Geometry check sheet. Reference: the model listing, model coordinates, mm. A direction names the side the tool comes from. Give positions to 0.01 mm unless a question says otherwise; leave off trailing zeros. Order: outer loops, then holes, each group sorted by start corner. A loop starts at its lowest first (then second) coordinate and runs counter-clockwise, first axis right, second up.
Autodesk Inventor part; units mm, degrees
ref_plane "ip_for_dummy_1_XY" through (0, 14.5, 0) normal (1, 0, 0) x (0, 0, -1)
ref_plane "ip_for_dummy_1_YZ" through (0, 14.5, 0) normal (0, 0, -1) x (0, 1, 0)
ref_plane "ip_for_dummy_1_ZX" through (0, 14.5, 0) normal (0, 1, 0) x (1, 0, 0)
sketch "Sketch_1" plane through (0, 0, 0) normal (1, 0, 0) x (0, 1, 0)
  line L0 (0, 18) -> (0, 2)
  arc A0 (0, 2) -> (2, 0) centre (2, 2) ccw
  line L1 (2, 0) -> (18, 0)
  line L2 (18, 0) -> (18, 1)
  line L3 (18, 1) -> (2, 1)
  arc A1 (1, 2) -> (2, 1) centre (2, 2) ccw
  line L4 (1, 2) -> (1, 18)
  line L5 (1, 18) -> (0, 18)
extrude "Extrusion1" add sketch "Sketch_1" along normal blind 52.5
sketch "Sketch_2" plane through (0, 0, 0) normal (0, 0, 1) x (1, 0, 0)
  arc A0 (1, 18) -> (0, 17) centre (1, 17) ccw
  line L0 (1, 18) -> (51.5, 18)
  arc A1 (52.5, 17) -> (51.5, 18) centre (51.5, 17) ccw
  line L1 (52.5, 17) -> (52.5, 23)
  line L2 (52.5, 23) -> (0, 23)
  line L3 (0, 23) -> (0, 17)
extrude "Extrusion2" cut sketch "Sketch_2" along normal blind 1
sketch "Sketch_3" plane through (0, 0, 0) normal (0, 1, 0) x (-1, 0, 0)
  line L0 (5, 0) -> (5, 23)
  line L1 (5, 23) -> (-57.5, 23)
  line L2 (-57.5, 23) -> (-57.5, 0)
  line L3 (-57.5, 0) -> (-52.5, 0)
  line L4 (-52.5, 0) -> (-52.5, 8.5)
  arc A0 (-51.5, 9.5) -> (-52.5, 8.5) centre (-51.5, 8.5) ccw
  line L5 (-51.5, 9.5) -> (-47.5, 9.5)
  arc A1 (-47, 9) -> (-47.5, 9.5) centre (-47.5, 9) ccw
  arc A2 (-47, 9) -> (-46.5, 8.5) centre (-46.5, 9) ccw
  line L6 (-46.5, 8.5) -> (-42.5, 8.5)
  arc A3 (-42.5, 8.5) -> (-42, 9) centre (-42.5, 9) ccw
  line L7 (-42, 9) -> (-42, 13)
  arc A4 (-42, 13) -> (-42.5, 13.5) centre (-42.5, 13) ccw
  line L8 (-42.5, 13.5) -> (-46.5, 13.5)
  arc A5 (-46.5, 13.5) -> (-47, 13) centre (-46.5, 13) ccw
  arc A6 (-47.5, 12.5) -> (-47, 13) centre (-47.5, 13) ccw
  line L9 (-47.5, 12.5) -> (-51.5, 12.5)
  arc A7 (-52.5, 13.5) -> (-51.5, 12.5) centre (-51.5, 13.5) ccw
  line L10 (-52.5, 13.5) -> (-52.5, 17)
  arc A8 (-51.5, 18) -> (-52.5, 17) centre (-51.5, 17) ccw
  line L11 (-51.5, 18) -> (-1, 18)
  arc A9 (0, 17) -> (-1, 18) centre (-1, 17) ccw
  line L12 (0, 17) -> (0, 13.5)
  arc A10 (-1, 12.5) -> (0, 13.5) centre (-1, 13.5) ccw
  line L13 (-1, 12.5) -> (-5, 12.5)
  arc A11 (-5.5, 13) -> (-5, 12.5) centre (-5, 13) ccw
  arc A12 (-5.5, 13) -> (-6, 13.5) centre (-6, 13) ccw
  line L14 (-6, 13.5) -> (-10, 13.5)
  arc A13 (-10, 13.5) -> (-10.5, 13) centre (-10, 13) ccw
  line L15 (-10.5, 13) -> (-10.5, 9)
  arc A14 (-10.5, 9) -> (-10, 8.5) centre (-10, 9) ccw
  line L16 (-10, 8.5) -> (-6, 8.5)
  arc A15 (-6, 8.5) -> (-5.5, 9) centre (-6, 9) ccw
  arc A16 (-5, 9.5) -> (-5.5, 9) centre (-5, 9) ccw
  line L17 (-5, 9.5) -> (-1, 9.5)
  arc A17 (0, 8.5) -> (-1, 9.5) centre (-1, 8.5) ccw
  line L18 (0, 8.5) -> (0, 0)
  line L19 (0, 0) -> (5, 0)
extrude "Extrusion3" cut sketch "Sketch_3" along normal blind 1
sketch "Sketch4" plane through (0, 0, 2) normal (0, -1, 0) x (1, 0, 0)
  point P0 (3.5, 5.5)
hole "Hole1" at (3.5, 0, 7.5) direction (0, 1, 0) diameter 2.46 depth 1
pattern_linear "Rectangular Pattern1" count 2 spacing 45.5 along (1, 0, 0) count 2 spacing 7 along (0, 0, 1) of "Hole1"
sketch "Sketch_6" plane through (4, 0, 0) normal (1, 0, 0) x (0, 0, -1)
  line L0 (5, 14.5) -> (-4, 14.5)
  line L1 (-4, 14.5) -> (-4, 16.95)
  arc A0 (-3.7, 17.25) -> (-4, 16.95) centre (-3.7, 16.95) ccw
  line L2 (-3.7, 17.25) -> (-1, 17.25)
  line L3 (-1, 17.25) -> (-1, 16)
  line L4 (-1, 16) -> (4.6935, 16)
  line L5 (4.6935, 16) -> (5, 15.6935)
  line L6 (5, 15.6935) -> (5, 14.5)
  line L7 (5, 14.5) -> (-4, 14.5)
revolve "Revolution1" add sketch "Sketch_6" angle 360 about axis through (4, 14.5, -5) along (0, 0, -1)
thread "Thread1"
pattern_linear "Rectangular Pattern2" count 2 spacing 44.5 along (1, 0, 0) of "Revolution1"
sketch "Sketch_8" plane through (0, 0, 4) normal (0, 0, 1) x (1, 0, 0)
  line L0 (2.75, 13.7783) -> (4, 13.0566)
  line L1 (4, 13.0566) -> (5.25, 13.7783)
  line L2 (5.25, 13.7783) -> (5.25, 15.2217)
  line L3 (5.25, 15.2217) -> (4, 15.9434)
  line L4 (4, 15.9434) -> (2.75, 15.2217)
  line L5 (2.75, 15.2217) -> (2.75, 13.7783)
extrude "Extrusion4" cut sketch "Sketch_8" against normal blind 1.3
pattern_linear "Rectangular Pattern3" count 2 spacing 44.5 along (1, 0, 0) of "Extrusion4"
ref_plane "ip_for_dummy_1_XY" through (0, 14.5, 0) normal (1, 0, 0) x (0, 0, -1)
ref_plane "ip_for_dummy_1_YZ" through (0, 14.5, 0) normal (0, 0, -1) x (0, 1, 0)
ref_plane "ip_for_dummy_1_ZX" through (0, 14.5, 0) normal (0, 1, 0) x (1, 0, 0)
ref_plane "ip_for_dummy_2_XY" through (52.5, 14.5, 0) normal (1, 0, 0) x (0, 0, -1)
ref_plane "ip_for_dummy_2_YZ" through (52.5, 14.5, 0) normal (0, 0, -1) x (0, 1, 0)
ref_plane "ip_for_dummy_2_ZX" through (52.5, 14.5, 0) normal (0, 1, 0) x (1, 0, 0)
ref_plane "ip_for_sensor_1_XY" through (0, 1, 11) normal (1, 0, 0) x (0, 0, -1)
ref_plane "ip_for_sensor_1_YZ" through (0, 1, 11) normal (0, 0, -1) x (0, 1, 0)
ref_plane "ip_for_sensor_1_ZX" through (0, 1, 11) normal (0, 1, 0) x (1, 0, 0)
ref_plane "ip_for_sensor_2_XY" through (52.5, 1, 11) normal (1, 0, 0) x (0, 0, -1)
ref_plane "ip_for_sensor_2_YZ" through (52.5, 1, 11) normal (0, 0, -1) x (0, 1, 0)
ref_plane "ip_for_sensor_2_ZX" through (52.5, 1, 11) normal (0, 1, 0) x (1, 0, 0)
properties part number "ETH2-14-sensor_plant"
Q1. Release check for a two-part mould opening along X. For faces 1 (the face through (52.5, 5.9, 0.8)), 2 (the face through (47.884, 15.588, 3.359)), 3 (the face through (49.116, 13.412, 3.359)), 4 (the face through (3, 0.5, 12.5)) record: pulls with the +X half, pulls with the -X half, needs draft (parallel to the pull), parting line crosses it, or undercut.
Q2. Gauge pin test, flat ends, axial feed: P1, Ø1, axis at x = 32.5, y = 15, coming from the +Z side; P2, Ø13, axis at x = 31, z = 11, coming from the +Y side; P3, Ø4, axis at x = 49, z = 14.5, coming from the -Y side; P4, Ø4, axis at x = 35, y = 11.5, coming from the -Z side. Record the tip position at first contact, or that the pin passes through.
Q3. Access from +Z, -Z, +X, -X, +Y, -Y to the whole of each face (thin tool, end or side, straight path). Record for faces 5 (the face through (25.882, 1.301, 1.285)), 6 (the face through (50.2, 0.51, 14.77)), 7 (the face through (47.25, 15, 3)), 8 (the face through (4, 13, -2)), 9 (the face through (52.215, 0.493, 9.199)).
Q4. Cross-section at B-B, the plane x = 25.5. Record the boundary of the cut face in (y, z), and give its area (3 significant figures).
Q5. Cross-section at A-A, the plane z = 7.5. Record the boundary of the cut face in (x, y), and give its area (3 significant figures).
Q6. Cross-section at C-C, the plane z = -3.25. Record the boundary of the cut face in (x, y), and give its area (3 significant figures).
Q7. Thickness scan on L1, parallel to X at y = 0.25, z = 7.5; L2, parallel to Z at x = 49, y = 0.2; L3, parallel to Z at x = 3.5, y = 0.3. Record the ranges inside material, lowest first.
Q8. Cross-section at D-D, the plane y = 3.5. Record the boundary of the cut face in (x, z), and give its area (3 significant figures).
Answers follow:
1. face 1: pulls with the +X half
1. face 2: undercut
1. face 3: undercut
1. face 4: needs draft
2. P1: stops at z = 1
2. P2: stops at y = 1
2. P3: stops at y = 0
2. P4: stops at z = 0
3. face 5: +Z, +X, -X
3. face 6: +Y, -Y
3. face 7: +Z
3. face 8: -Z
3. face 9: +X, +Y, -Y
4. outline: (0, 2) arc R2 ccw to (2, 0) - (18, 0) - (18, 1) - (2, 1) arc R1 cw to (1, 2) - (1, 18) - (0, 18) - close
4. area: 34.4 mm2
5. outline: (0, 0) - (2.27, 0) - (2.27, 1) - (0, 1) - close; (4.73, 0) - (47.77, 0) - (47.77, 1) - (4.73, 1) - close; (50.23, 0) - (52.5, 0) - (52.5, 1) - (50.23, 1) - close
5. area: 47.6 mm2
6. outline: circle Ø3 at (4, 14.5); circle Ø3 at (48.5, 14.5)
6. area: 14.1 mm2
7. L1: x = 0 to 2.27, 4.73 to 47.77, 50.23 to 52.5
7. L2: z = 1.13 to 6.27, 8.73 to 9.5, 12.5 to 13.27, 15.73 to 18
7. L3: z = 0.95 to 6.27, 8.73 to 9.5, 12.5 to 13.27, 15.73 to 18
8. outline: (0, 0) - (52.5, 0) - (52.5, 1) - (0, 1) - close
8. area: 52.5 mm2
